from build123d import *

# Parameters (mm, degrees)
F0_W      = 31.75
F0_H      = 63.5
F1_DEPTH  = 7.62
F2_W      = 11.7348
F2_H      = 7.62
F3_DEPTH  = 19.05
F4_W      = 13.97
F4_H      = 7.62
F5_DEPTH  = 33.02
F6_W      = 13.97
F6_H      = 7.62
F7_DEPTH  = 33.02
F8_R      = 2.159
F8_W      = 0.508
F8_H      = 7.62
F8_W_2    = 2.54
F9_DEPTH  = 7.621
F10_DEPTH = 10.0076
F11_DEPTH = 10.0076
F8_W_3    = 10.922
F12_DEPTH = 3.81
F13_DEPTH = 8.75000028
F14_DEPTH = 8.75000028
F15_DEPTH = 6.477
F16_W     = 18.51600056
F16_H     = 5.08
F17_DEPTH = 35.56


with BuildPart() as f1:
    # F0 (on Top) → F1 (new body)
    with BuildSketch(Plane.XY):
        with Locations((15.875, -31.75)):
            Rectangle(F0_W, F0_H)
    extrude(amount=F1_DEPTH)

    # F2 (on face) → F3 (join)
    with BuildSketch(Plane.XZ.offset(63.5)):
        with Locations((15.875, 3.81)):
            Rectangle(F2_W, F2_H)
    extrude(amount=F3_DEPTH)

    # F4 (on face) → F5 (join)
    with BuildSketch(Plane(origin=(10.0076, 0, 0), x_dir=(0, -1, 0), z_dir=(-1, 0, 0))):
        with Locations((75.565, 3.81)):
            Rectangle(F4_W, F4_H)
    extrude(amount=F5_DEPTH)

    # F6 (on face) → F7 (join)
    with BuildSketch(Plane.YZ.offset(21.7424)):
        with Locations((-75.565, 3.81)):
            Rectangle(F6_W, F6_H)
    extrude(amount=F7_DEPTH)

    # F8 (on face) → F9 (cut, through all)
    with BuildSketch(Plane.XY.offset(7.62)):
        with Locations((49.0474, -75.565)):
            Circle(F8_R)
        Polygon((37.6174, -71.755), (40.1574, -71.755), (40.6654, -71.755), (40.6654, -71.247), (37.1094, -71.247), (37.1094, -79.883), (40.6654, -79.883), (40.6654, -79.375), (40.1574, -79.375), (37.6174, -79.375), align=None)
        with Locations((40.4114, -75.565)):
            Rectangle(F8_W, F8_H)
        with Locations((38.8874, -75.565)):
            Rectangle(F8_W_2, F8_H)
        with Locations((-17.2974, -75.565)):
            Circle(F8_R)
        Polygon((-8.4074, -71.755), (-5.8674, -71.755), (-5.8674, -79.375), (-8.4074, -79.375), (-8.9154, -79.375), (-8.9154, -79.883), (-5.3594, -79.883), (-5.3594, -71.247), (-8.9154, -71.247), (-8.9154, -71.755), align=None)
        with Locations((-8.6614, -75.565)):
            Rectangle(F8_W, F8_H)
        with Locations((-7.1374, -75.565)):
            Rectangle(F8_W_2, F8_H)
    extrude(amount=-F9_DEPTH, mode=Mode.SUBTRACT)

    # F10 (add): a face of the model
    f10_faces = [f1.faces().sort_by_distance(p)[0] for p in [
        (10.0076, -66.04, 3.81),
    ]]
    extrude(f10_faces, amount=F10_DEPTH)

    # F11 (add): a face of the model
    f11_faces = [f1.faces().sort_by_distance(p)[0] for p in [
        (21.7424, -66.04, 3.81),
    ]]
    extrude(f11_faces, amount=F11_DEPTH)

    # F8 (on face) → F12 (cut)
    with BuildSketch(Plane.XY.offset(7.62)):
        with Locations((46.1264, -75.565)):
            Rectangle(F8_W_3, F8_H)
        with Locations((49.0474, -75.565)):
            Circle(F8_R, mode=Mode.SUBTRACT)
        Polygon((40.6654, -71.247), (40.6654, -71.755), (51.5874, -71.755), (51.5874, -79.375), (40.6654, -79.375), (40.6654, -79.883), (52.0954, -79.883), (52.0954, -71.247), align=None)
        with Locations((-14.3764, -75.565)):
            Rectangle(F8_W_3, F8_H)
        with Locations((-17.2974, -75.565)):
            Circle(F8_R, mode=Mode.SUBTRACT)
        Polygon((-19.8374, -71.755), (-8.9154, -71.755), (-8.9154, -71.247), (-20.3454, -71.247), (-20.3454, -79.883), (-8.9154, -79.883), (-8.9154, -79.375), (-19.8374, -79.375), align=None)
    extrude(amount=-F12_DEPTH, mode=Mode.SUBTRACT)

    # F13 (add): a face of the model
    f13_faces = [f1.faces().sort_by_distance(p)[0] for p in [
        (0, -34.29, 3.81),
    ]]
    extrude(f13_faces, amount=F13_DEPTH)

    # F14 (add): a face of the model
    f14_faces = [f1.faces().sort_by_distance(p)[0] for p in [
        (31.75, -34.29, 3.81),
    ]]
    extrude(f14_faces, amount=F14_DEPTH)

    # F15 (add): a face of the model
    f15_faces = [f1.faces().sort_by_distance(p)[0] for p in [
        (15.875, 0, 3.81),
    ]]
    extrude(f15_faces, amount=F15_DEPTH)

    # F16 (on face) → F17 (join)
    with BuildSketch(Plane(origin=(0, 0, 0), x_dir=(1, 0, 0), z_dir=(0, 0, -1))):
        with Locations((15.875, -3.937)):
            Rectangle(F16_W, F16_H)
        with Locations((15.875, 80.01)):
            Rectangle(F16_W, F16_H)
        Polygon((2.80699972, -6.477), (6.61699972, -6.477), (6.61699972, -1.397), (6.61699972, 77.47), (6.61699972, 82.55), (2.80699972, 82.55), align=None)
        Polygon((25.13300028, -1.397), (25.13300028, -6.477), (28.94300028, -6.477), (28.94300028, 82.55), (25.13300028, 82.55), (25.13300028, 77.47), align=None)
    extrude(amount=F17_DEPTH)


solid = f1.part
Geometry: final body of the model. Coordinates: model frame, mm. A direction names the side the tool comes from. Coordinates: 2 decimals unless noted, no trailing zeros. Loops run counter-clockwise (first coordinate to the right, second up) from the corner with the lowest first, then second, coordinate; pieces in that order, holes last. Notation, with made-up numbers: M 26.5,67 L 60.5,67 A20 cw 60.5,86 Z; hole C 89.25,75 d5. An arc over 180 degrees is marked long. One line per item, written item: value. Start each with the question number.
1) Cut plane B-B (x = 12). Return loops of the section in (y, z).
2) Material intervals for L1, parallel to X at y = -3, z = -12; L2, parallel to X at y = -72, z = 4.5; L3, parallel to Y at x = 23, z = -23, sorted ascending. Write a range as from..to.
3) Cut plane C-C (y = -23). Return loops of the section in (x, z), then the cut area to 3 significant figures.
4) Reachability of faces 4 (the flat face through (16, -77.47, -18)), 5 (the flat face through (40.665, -76, 2)), 6 (the flat face through (48, -68.58, 4)), 7 (the flat face through (-4, -39, 0)) from +Z, -Z, +X, -X, +Y, -Y: full face, straight path, thin tool, end or side. Return the list, or none.
5) Cut plane A-A (z = -13). Return loops of the section in (x, y).
6) Cut plane D-D (x = 44.5). Return loops of the section in (y, z).
7) Pin query (flat end, axial travel): P1, Ø8, axis at y = -42.5, z = -30, coming from the +X side; P2, Ø9.5, axis at x = 17.5, y = -47, coming from the -Z side; P3, Ø1.5, axis at y = -44.5, z = 2.5, coming from the +X side; P4, Ø3, axis at x = -11, y = -31.5, coming from the +Z side. Return the tip coordinate at first contact, or that it passes through.
8) Draft query along X for faces 1 (the flat face through (16, 6.477, -9)), 2 (the flat face through (-5.359, -76, 4)), 3 (the flat face through (2.807, -39, -18)). Return one class per face: released by +X, released by -X, zero draft, split by the parting line, or undercut.
Evaluation:
1. outline: M -82.55,-35.56 L -77.47,-35.56 L -77.47,0 L 1.4,0 L 1.4,-35.56 L 6.48,-35.56 L 6.48,7.62 L -82.55,7.62 Z
2. L1: 2.81..6.62, 25.13..28.94
2. L2: -23.01..-20.35, -5.36..37.11, 52.1..54.76
2. L3: -82.55..-77.47, 1.4..6.48
3. outline: M -8.75,0 L 2.81,0 L 2.81,-35.56 L 6.62,-35.56 L 6.62,0 L 25.13,0 L 25.13,-35.56 L 28.94,-35.56 L 28.94,0 L 40.5,0 L 40.5,7.62 L -8.75,7.62 Z
3. area: 646 mm^2
4. face 4: -Z
4. face 5: +Z, -Z
4. face 6: +Z, -Z, +X, +Y
4. face 7: -Z, -X, +Y, -Y
5. outline: M 2.81,-82.55 L 28.94,-82.55 L 28.94,6.48 L 2.81,6.48 Z; hole M 6.62,-77.47 L 25.13,-77.47 L 25.13,1.4 L 6.62,1.4 Z
6. outline: M -82.55,0 L -68.58,0 L -68.58,7.62 L -71.25,7.62 L -71.25,3.81 L -79.88,3.81 L -79.88,7.62 L -82.55,7.62 Z
7. P1: x = 28.94
7. P2: z = 0
7. P3: x = 40.5
7. P4: through
8. face 1: zero draft
8. face 2: undercut
8. face 3: released by -X
